Could you check a few things on this model? Use its own coordinates, in mm. Coordinates: 2 decimals unless noted, no trailing zeros. Write each loop counter-clockwise with the first axis right and the second up, starting at its lowest first coordinate (ties: lowest second). Pieces come first, ordered by that corner, then holes. Notation, with made-up numbers: (-18, 30.25) - (9, 30.25) arc R26 cw to (9, 62.25) - close; hole circle Ø5 at (44, 26.25). An arc over 180 degrees is marked (long way). Write item = value, one per line. Start each with the question number.
Autodesk Inventor part; units mm, degrees
ref_plane "YZ Plane" through (0, 0, 0) normal (1, 0, 0) x (0, 1, 0)
ref_plane "XZ Plane" through (0, 0, 0) normal (0, 1, 0) x (-1, 0, 0)
ref_plane "XY Plane" through (0, 0, 0) normal (0, 0, 1) x (1, 0, 0)
sketch "草圖5" plane through (0, 0, 0) normal (0, 0, 1) x (1, 0, 0)
  line L0 (-110, -110) -> (110, -110)
  line L1 (110, -110) -> (110, 110)
  line L2 (110, 110) -> (-110, 110)
  line L3 (-110, 110) -> (-110, -110)
  line L4 (-110, -110) -> (110, 110) construction
  line L5 (110, -110) -> (-110, 110) construction
  circle A0 centre (0, 0) radius 13.25
  dimension "d29" = 220
  dimension "d30" = 220
  dimension "d33" = 26.5
extrude "擠出6" add sketch "草圖5" along normal mid plane 340
equation "\"th6\" = T1A_th6"
equation "\"T1A_th6\" = 45deg"
equation "\"T1A_R1\" = 585.5331"
equation "\"T1A_R3\" = 252.3048"
equation "\"T1A_R4\" = 320.6953"
equation "\"T1A_R5\" = 419.3047"
equation "\"T1A_R7\" = -221.7475"
equation "\"T1A_R8\" = 369.2781"
equation "\"T1A_R1_Width\" = 756"
equation "\"T1A_R2_Width\" = 756"
equation "\"T1A_R3_Width\" = 344"
equation "\"T1A_R4_Width\" = 756"
equation "\"T1A_Joint_Width\" = 756"
properties part number "Type 1A R6主滑台:1" material "密度7850的鋼"
1) Suppose I cut it at A-A on y = 0. Please give me the cut outline in (x, z), plus the area to 3 significant figures.
2) Thinking about a two-plate mould opening in Y: for faces 1 (the flat face through (-2, 26, 170)), 2 (the cylindrical face through (7.123, -11.172, -2.38)), 3 (the flat face through (-2, -110, -2)), which applies, +Y half, -Y half, draft (parallel to the pull), parting line (faces both ways), or undercut?
3) If I drill on probe 1 along Y at (x, z) = (0, 59), over which ranges is the centre line in solid material (lowest first)? Write a range as [from, to].
Reply:
q1.outline = (-110, -170) - (-13.25, -170) - (-13.25, 170) - (-110, 170) - close; (13.25, -170) - (110, -170) - (110, 170) - (13.25, 170) - close
q1.area = 65,800 mm^2
q2.face_1 = draft
q2.face_2 = undercut
q2.face_3 = -Y half
q3.probe_1 = [-110, -13.25], [13.25, 110]
